Geometry check sheet. Reference: the model listing, model coordinates, mm. Face numbers are marked on the shaded views. A direction names the side the tool comes from. Coordinates: 2 decimals unless noted, no trailing zeros. Write each loop counter-clockwise with the first axis right and the second up, starting at its lowest first coordinate (ties: lowest second). Pieces come first, ordered by that corner, then holes. Notation, with made-up numbers: (-36, 60) -> (8, 60) arc R24 cw to (8, 92) -> close; hole circle Ø7 at (48, 33). An arc over 180 degrees is marked (long way). Answer in a Markdown table with one row per item. Add a question column.
1. Scan lines: L1, parallel to X at y = 19.5, z = 18.75; L2, parallel to Y at x = -19, z = 17; L3, parallel to X at y = 20.5, z = 3.75. Record each from-to range of solid material in increasing order. Write a range as from..to.
2. Cross-section at A-A on x = -15.5. Record the cut outline in (y, z), and give its area (3 significant figures).
3. Mould release check, pull along Y, two halves, no side actions. Record for the marked faces 4 and 5: pulls with the +Y half, pulls with the -Y half, needs draft (parallel to the pull), parting line crosses it, or undercut.
4. Set-up check for the marked faces 1, 2 and 3: record each of +Z, -Z, +X, -X, +Y, -Y from which the full face is reachable in a straight line by a thin tool's end or side.
5. Depth check by flat-ended pin: P1, Ø13, axis at x = -10.5, y = 2.5, coming from the +Z side; P2, Ø4, axis at y = 0.5, z = 1, coming from the -X side; P3, Ø5, axis at x = -11.5, z = 7, coming from the -Y side; P4, Ø10, axis at y = 6, z = 16, coming from the +X side. Enter the tip coordinate at first touch or a pass-through.
6. Cross-section at C-C on y = -16. Record the cut outline in (x, z).
7. Cross-section at B-B on z = 11. Record the cut outline in (x, y).
Autodesk Fusion 360 part; units mm, degrees
sketch "草图1" plane through (0, 0, 0) normal (0, 0, 1) x (1, 0, 0) in component "spinner with 4 wheel v3"
  circle A0 centre (-19.1272, 19.1272) radius 4.95
  circle A1 centre (19.1272, 19.1272) radius 4.95
  circle A2 centre (19.1272, -19.1272) radius 4.95
  circle A3 centre (-19.1272, -19.1272) radius 4.95
  ellipse E0 centre (32, 0) end of major axis (47, 0) minor radius 20.5 (21.6933, 14.8943) -> (21.6933, -14.8943) ccw
  ellipse E1 centre (0, 32) end of major axis (0, 47) minor radius 20.5 (-14.8943, 21.6933) -> (14.8943, 21.6933) ccw
  line L0 (0, 41) -> (0, 70)
  line L1 (0, -47) -> (0, -70)
  ellipse E2 centre (-32, 0) end of major axis (-17, 0) minor radius 20.5 (-21.6933, -14.8943) -> (-21.6933, 14.8943) ccw
  ellipse E3 centre (0, -32) end of major axis (0, -17) minor radius 20.5 (14.8943, -21.6933) -> (-14.8943, -21.6933) ccw
  line L2 (3.25, 1.8764) -> (0, 3.7528)
  line L3 (0, 3.7528) -> (-3.25, 1.8764)
  line L4 (-3.25, 1.8764) -> (-3.25, -1.8764)
  line L5 (-3.25, -1.8764) -> (0, -3.7528)
  line L6 (0, -3.7528) -> (3.25, -1.8764)
  line L7 (3.25, -1.8764) -> (3.25, 1.8764)
  line L8 (30, -20) -> (19.1272, -19.1272)
  dimension "d5" = 9.9
  dimension "d6" = 9.9
  dimension "d7" = 9.9
  dimension "d8" = 9.9
  dimension "d9" = 30
  dimension "d10" = 41
  dimension "d15" = 30
  dimension "d16" = 41
  dimension "d17" = 3.25
extrude "拉伸1" add sketch "草图1" along normal blind 5 in component "spinner with 4 wheel v3"
sketch "草图2" plane through (0, 0, 5) normal (0, 0, 1) x (-1, 0, 0) in component "spinner with 4 wheel v3"
  line L0 (-3.25, -1.8764) -> (-3.25, 1.8764)
  line L1 (-3.25, 1.8764) -> (0, 3.7528)
  line L2 (0, 3.7528) -> (3.25, 1.8764)
  line L3 (3.25, 1.8764) -> (3.25, -1.8764)
  line L4 (3.25, -1.8764) -> (0, -3.7528)
  line L5 (0, -3.7528) -> (-3.25, -1.8764)
  ellipse E0 centre (0, 32) end of major axis (20.5, 32) minor radius 15 (-14.8943, 21.6933) -> (14.8943, 21.6933) ccw
  arc A0 (-14.8943, 21.6933) -> (-21.6933, 14.8943) centre (-19.1272, 19.1272) ccw
  ellipse E1 centre (-32, 0) end of major axis (-32, -20.5) minor radius 15 (-21.6933, -14.8943) -> (-21.6933, 14.8943) ccw
  arc A1 (-21.6933, -14.8943) -> (-14.8943, -21.6933) centre (-19.1272, -19.1272) ccw
  ellipse E2 centre (0, -32) end of major axis (20.5, -32) minor radius 15 (14.8943, -21.6933) -> (-14.8943, -21.6933) ccw
  arc A2 (14.8943, -21.6933) -> (21.6933, -14.8943) centre (19.1272, -19.1272) ccw
  ellipse E3 centre (32, 0) end of major axis (32, -20.5) minor radius 15 (21.6933, 14.8943) -> (21.6933, -14.8943) ccw
  arc A3 (21.6933, 14.8943) -> (14.8943, 21.6933) centre (19.1272, 19.1272) ccw
  circle A4 centre (-19.1272, -19.1272) radius 4.95
  circle A5 centre (19.1272, -19.1272) radius 4.95
  circle A6 centre (19.1272, 19.1272) radius 4.95
  circle A7 centre (-19.1272, 19.1272) radius 4.95
  dimension "d20" = 9.9
  dimension "d21" = 4.95
  dimension "d22" = 9.9
  dimension "d23" = 4.95
extrude "拉伸2" add sketch "草图2" along normal blind 7 contours A0 A7 | A3 A6 | A1 A4 | A2 A5 in component "spinner with 4 wheel v3"
sketch "草图3" plane through (0, 0, 5) normal (0, 0, 1) x (-1, 0, 0) in component "spinner with 4 wheel v3"
  arc A0 (-14.8943, -21.6933) -> (-21.6933, -14.8943) centre (-19.1272, -19.1272) ccw
  ellipse E0 centre (0, -32) end of major axis (20.5, -32) minor radius 15 (14.8943, -21.6933) -> (-14.8943, -21.6933) ccw
  arc A1 (21.6933, -14.8943) -> (14.8943, -21.6933) centre (19.1272, -19.1272) ccw
  ellipse E1 centre (32, 0) end of major axis (32, -20.5) minor radius 15 (21.6933, 14.8943) -> (21.6933, -14.8943) ccw
  arc A2 (14.8943, 21.6933) -> (21.6933, 14.8943) centre (19.1272, 19.1272) ccw
  ellipse E2 centre (0, 32) end of major axis (20.5, 32) minor radius 15 (-14.8943, 21.6933) -> (14.8943, 21.6933) ccw
  arc A3 (-21.6933, 14.8943) -> (-14.8943, 21.6933) centre (-19.1272, 19.1272) ccw
  ellipse E3 centre (-32, 0) end of major axis (-32, -20.5) minor radius 15 (-21.6933, -14.8943) -> (-21.6933, 14.8943) ccw
  line L0 (-3.25, -1.8764) -> (-3.25, 1.8764)
  line L1 (-3.25, 1.8764) -> (0, 3.7528)
  line L2 (0, 3.7528) -> (3.25, 1.8764)
  line L3 (3.25, 1.8764) -> (3.25, -1.8764)
  line L4 (3.25, -1.8764) -> (0, -3.7528)
  line L5 (0, -3.7528) -> (-3.25, -1.8764)
  line L6 (-3.25, -1.8764) -> (0, -3.7528)
  line L7 (0, -3.7528) -> (3.25, -1.8764)
  line L8 (3.25, -1.8764) -> (3.25, 1.8764)
  line L9 (3.25, 1.8764) -> (0, 3.7528)
  line L10 (0, 3.7528) -> (-3.25, 1.8764)
  line L11 (-3.25, 1.8764) -> (-3.25, -1.8764)
extrude "拉伸3" add sketch "草图3" against normal blind 2 contours L0 L1 L2 L3 L4 L5 L6 L7 L8 L9 L10 L11 in component "spinner with 4 wheel v3"
sketch "草图4" plane through (0, 0, 5) normal (0, 0, 1) x (-1, 0, 0) in component "spinner with 4 wheel v3"
  arc A0 (-14.8943, -21.6933) -> (-21.6933, -14.8943) centre (-19.1272, -19.1272) ccw
  ellipse E0 centre (0, -32) end of major axis (20.5, -32) minor radius 15 (14.8943, -21.6933) -> (-14.8943, -21.6933) ccw
  arc A1 (21.6933, -14.8943) -> (14.8943, -21.6933) centre (19.1272, -19.1272) ccw
  ellipse E1 centre (32, 0) end of major axis (32, -20.5) minor radius 15 (21.6933, 14.8943) -> (21.6933, -14.8943) ccw
  arc A2 (14.8943, 21.6933) -> (21.6933, 14.8943) centre (19.1272, 19.1272) ccw
  ellipse E2 centre (0, 32) end of major axis (20.5, 32) minor radius 15 (-14.8943, 21.6933) -> (14.8943, 21.6933) ccw
  arc A3 (-21.6933, 14.8943) -> (-14.8943, 21.6933) centre (-19.1272, 19.1272) ccw
  ellipse E3 centre (-32, 0) end of major axis (-32, -20.5) minor radius 15 (-21.6933, -14.8943) -> (-21.6933, 14.8943) ccw
  circle A4 centre (0, 0) radius 2
extrude "拉伸4" add sketch "草图4" along normal blind 15 contours A4 in component "spinner with 4 wheel v3"
sketch "草图5" plane through (0, 0, 0) normal (0, 0, 1) x (1, 0, 0) in component "spinner with 4 wheel v3"
extrude "拉伸5" add 1 faces at (1.0833, -0.6255, 3) along direction (0, 0, -1) blind 3 in component "spinner with 4 wheel v3"
sketch "草图6" plane through (0, 0, 0) normal (0, 0, 1) x (1, 0, 0) in component "spinner with 4 wheel v3"
  line L0 (-3.2, -1.8475) -> (0, -3.695)
  line L1 (0, -3.695) -> (3.2, -1.8475)
  line L2 (3.2, -1.8475) -> (3.2, 1.8475)
  line L3 (3.2, 1.8475) -> (0, 3.695)
  line L4 (0, 3.695) -> (-3.2, 1.8475)
  line L5 (-3.2, 1.8475) -> (-3.2, -1.8475)
  dimension "d32" = 3.2
extrude "拉伸6" cut sketch "草图6" along normal blind 22 in component "spinner with 4 wheel v3"
sketch "草图7" plane through (0, 0, 0) normal (1, 0, 0) x (0, 1, 0) in component "spinner with 4 wheel v3"
extrude "拉伸7" cut 4 faces at (18.1573, 20.0862, 12) (16.979, -18.0927, 12) (-17.5166, -19.4446, 12) (-20.5586, 20.6052, 12) along direction (0, 0, -1) blind 12 in component "spinner with 4 wheel v3"
sketch "草图8" plane through (0, 0, 5) normal (0, 0, 1) x (-1, 0, 0) in component "spinner with 4 wheel v3"
  arc A0 (-14.8943, -21.6933) -> (-21.6933, -14.8943) centre (-19.1272, -19.1272) ccw
  ellipse E0 centre (0, -32) end of major axis (20.5, -32) minor radius 15 (14.8943, -21.6933) -> (-14.8943, -21.6933) ccw
  arc A1 (21.6933, -14.8943) -> (14.8943, -21.6933) centre (19.1272, -19.1272) ccw
  ellipse E1 centre (32, 0) end of major axis (32, -20.5) minor radius 15 (21.6933, 14.8943) -> (21.6933, -14.8943) ccw
  arc A2 (14.8943, 21.6933) -> (21.6933, 14.8943) centre (19.1272, 19.1272) ccw
  ellipse E2 centre (0, 32) end of major axis (20.5, 32) minor radius 15 (-14.8943, 21.6933) -> (14.8943, 21.6933) ccw
  arc A3 (-21.6933, 14.8943) -> (-14.8943, 21.6933) centre (-19.1272, 19.1272) ccw
  ellipse E3 centre (-32, 0) end of major axis (-32, -20.5) minor radius 15 (-21.6933, -14.8943) -> (-21.6933, 14.8943) ccw
  circle A4 centre (-19.1272, 19.1272) radius 5
  circle A5 centre (-19.1272, -19.1272) radius 5
  circle A6 centre (19.1272, 19.1272) radius 5
  circle A7 centre (19.1272, -19.1272) radius 5
  line L0 (3.2, -1.8475) -> (0, -3.695)
  line L1 (0, -3.695) -> (-3.2, -1.8475)
  line L2 (-3.2, -1.8475) -> (-3.2, 1.8475)
  line L3 (-3.2, 1.8475) -> (0, 3.695)
  line L4 (0, 3.695) -> (3.2, 1.8475)
  line L5 (3.2, 1.8475) -> (3.2, -1.8475)
  dimension "d37" = 4.95
  dimension "d38" = 4.95
  dimension "d39" = 4.95
  dimension "d40" = 4.95
  dimension "d41" = 10
  dimension "d42" = 10
  dimension "d43" = 10
  dimension "d44" = 10
extrude "拉伸8" add sketch "草图8" along normal blind -5 and the other way blind -7 contours A0 E0 E3 A5 | A0 E0 E3 A5 | E0 A1 E1 A7 | E0 A1 E1 A7 | E2 A3 E3 A4 | E2 A3 E3 A4 | E1 A2 E2 A6 | E1 A2 E2 A6 in component "spinner with 4 wheel v3"
extrude "拉伸9" add 4 faces at (20.5783, 17.6971, 12) (-17.6037, 17.7136, 12) (-20.6618, -20.4674, 12) (18.5183, -20.4625, 12) along direction (0, 0, 1) blind 8 in component "spinner with 4 wheel v3"
extrude "拉伸10" add 1 faces at (9.8129, -9.3621, 0) along direction (0, 0, -1) blind 5 in component "spinner with 4 wheel v3"
sketch "草图1 (2)" plane through (0, 0, 0) normal (1, 0, 0) x (0, 1, 0)
component "spinner with 4 wheel v3" placed x (1, 0, 0) y (0, 1, 0) z (0, 0, 1) at (0, 0, 0)
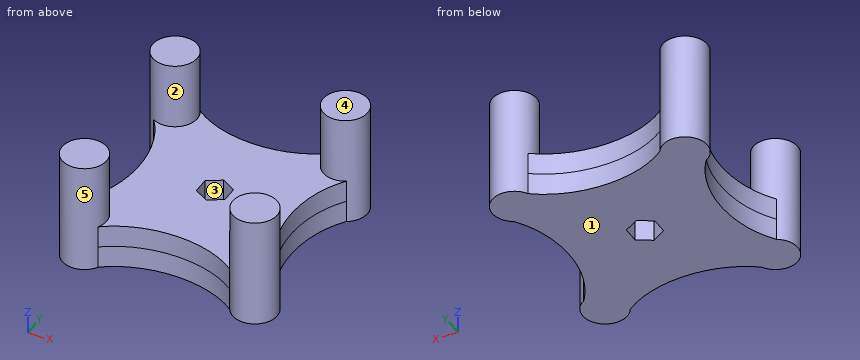
Results found:
| question | item | result |
|---|---|---|
| 1 | L1 | x = -24.11..-14.14, 14.14..24.11 |
| 1 | L2 | y = -24.13..-14.13, 14.13..24.13 |
| 1 | L3 | x = -23.94..-13.16, 13.16..23.94 |
| 2 | outline | (-22.57, -5) -> (22.57, -5) -> (22.57, 20) -> (15.69, 20) -> (15.69, 5) -> (-15.69, 5) -> (-15.69, 20) -> (-22.57, 20) -> close |
| 2 | area | 658 mm^2 |
| 3 | face 4 | needs draft |
| 3 | face 5 | undercut |
| 4 | face 1 | -Z, +X, -X, +Y, -Y |
| 4 | face 2 | +Z |
| 4 | face 3 | +Z, -Z |
| 5 | P1 | stops at z = 5 |
| 5 | P2 | stops at x = -17.11 |
| 5 | P3 | stops at y = -20.4 |
| 5 | P4 | passes through |
| 6 | outline | (-23.03, -5) -> (23.03, -5) -> (23.03, 20) -> (15.23, 20) -> (15.23, 5) -> (-15.23, 5) -> (-15.23, 20) -> (-23.03, 20) -> close |
| 7 | outline | circle Ø10 at (-19.13, -19.13); circle Ø10 at (-19.13, 19.13); circle Ø10 at (19.13, -19.13); circle Ø10 at (19.13, 19.13) |
